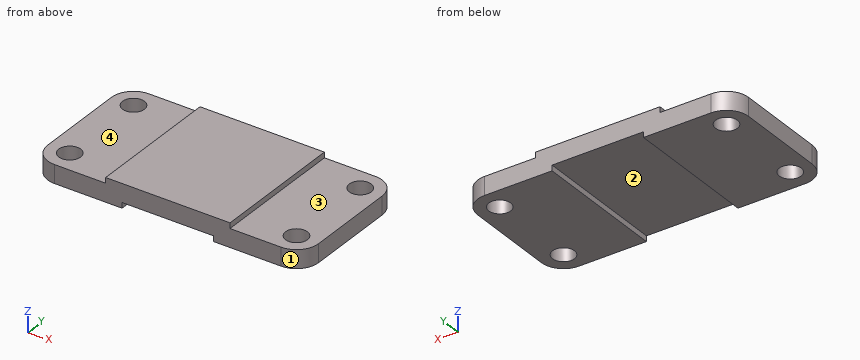
```python
from build123d import *

# Parameters (mm, degrees)
F1_DEPTH = 37
F2_R     = 12
F3_R     = 6
F4_DEPTH = 25


# Not quite as in the source:
# - a pattern or mirror of a feature is missing from the dataset's text; its kind, count and spacing are read off the source's solid


with BuildPart() as f1:
    # F0 (on Front) → F1 (new body, symmetric)
    with BuildSketch(Plane.XZ):
        Polygon((-25, 3), (0, 3), (25, 3), (25, 0), (74, 0), (74, 10), (34, 10), (34, 13), (0, 13), (-34, 13), (-34, 10), (-74, 10), (-74, 0), (-25, 0), align=None)
    extrude(amount=F1_DEPTH, both=True)

    # F2
    f2_edges = [f1.edges().sort_by_distance(p)[0] for p in [
        (74, -37, 5),
        (74, 37, 5),
        (-74, -37, 5),
        (-74, 37, 5),
    ]]
    fillet(f2_edges, radius=F2_R)

    # F3 (on face) → F4 (cut)
    with BuildSketch(Plane.XY.offset(10)):
        with Locations((-62, -25)):
            Circle(F3_R)
    f4 = extrude(amount=-F4_DEPTH, mode=Mode.SUBTRACT)

    # F4_copies: F4 across plane
    add(f4.mirror(Plane.ZX), mode=Mode.SUBTRACT)

    # F4_copies1: F4 across plane
    add(f4.mirror(Plane(origin=(0, 0, 0), x_dir=(-0.3739683355, 0.927441472, 0), z_dir=(0.927441472, 0.3739683355, 0))), mode=Mode.SUBTRACT)

    # F4_copies2: F4 across plane
    add(f4.mirror(Plane(origin=(0, 0, 0), x_dir=(0, 0, 1), z_dir=(1, 0, 0))), mode=Mode.SUBTRACT)


solid = f1.part
```
Check sheet for the modelled part. Datum: model origin and axes. Units: mm. Face numbers are marked on the shaded views. A direction names the side the tool comes from. Coordinates: 2 decimals unless noted, no trailing zeros. Loops run counter-clockwise (first coordinate to the right, second up) from the corner with the lowest first, then second, coordinate; pieces in that order, holes last.
1) Material ranges on probe 1 along Y at (x, z) = (62, 3.75); probe 2 along X at (y, z) = (-28, 4.5); probe 3 along X at (y, z) = (30.5, 2.5), recorded low to high.
2) Sectioned sample at D-D (x = 54). Record the boundary of the cut face in (y, z), and give its area (3 significant figures).
3) Sectioned sample at C-C (y = -3). Record the boundary of the cut face in (x, z).
4) Sectioned sample at B-B (x = -59). Record the boundary of the cut face in (y, z).
5) Gauge pin test, flat ends, axial feed: pin 1 (25 mm diameter, centred on x = 5.5, y = 15, fed in from -Z); pin 2 (20 mm diameter, centred on x = 50.5, y = 11.5, fed in from +Z); pin 3 (2.5 mm diameter, centred on y = -5, z = 12, fed in from +X); pin 4 (7 mm diameter, centred on x = 62, y = -25, fed in from -Z). Record the tip position at first contact, or that the pin passes through.
6) Access from +Z, -Z, +X, -X, +Y, -Y to the whole of each face (thin tool, end or side, straight path). Record for the marked faces 1, 2, 3 and 4.
7) Sectioned sample at A-A (y = -29.5). Record the boundary of the cut face in (x, z).
Check sheet entries:
1. probe 1: y = -37 to -31, -19 to 19, 31 to 37
1. probe 2: x = -73.62 to -67.2, -56.8 to 56.8, 67.2 to 73.62
1. probe 3: x = -72.67 to -64.4, -59.6 to -25, 25 to 59.6, 64.4 to 72.67
2. outline: (-37, 0) - (37, 0) - (37, 10) - (-37, 10) - close
2. area: 740 mm2
3. outline: (-74, 0) - (-25, 0) - (-25, 3) - (25, 3) - (25, 0) - (74, 0) - (74, 10) - (34, 10) - (34, 13) - (-34, 13) - (-34, 10) - (-74, 10) - close
4. outline: (-37, 0) - (-30.2, 0) - (-30.2, 10) - (-37, 10) - close; (-19.8, 0) - (19.8, 0) - (19.8, 10) - (-19.8, 10) - close; (30.2, 0) - (37, 0) - (37, 10) - (30.2, 10) - close
5. pin 1: stops at z = 3
5. pin 2: stops at z = 10
5. pin 3: stops at x = 34
5. pin 4: passes through
6. face 1: +Z, -Z, +X, -Y
6. face 2: -Z, +Y, -Y
6. face 3: +Z, +X, +Y, -Y
6. face 4: +Z, -X, +Y, -Y
7. outline: (-73.12, 0) - (-65.97, 0) - (-65.97, 10) - (-73.12, 10) - close; (-58.03, 0) - (-25, 0) - (-25, 3) - (25, 3) - (25, 0) - (58.03, 0) - (58.03, 10) - (34, 10) - (34, 13) - (-34, 13) - (-34, 10) - (-58.03, 10) - close; (65.97, 0) - (73.12, 0) - (73.12, 10) - (65.97, 10) - close
